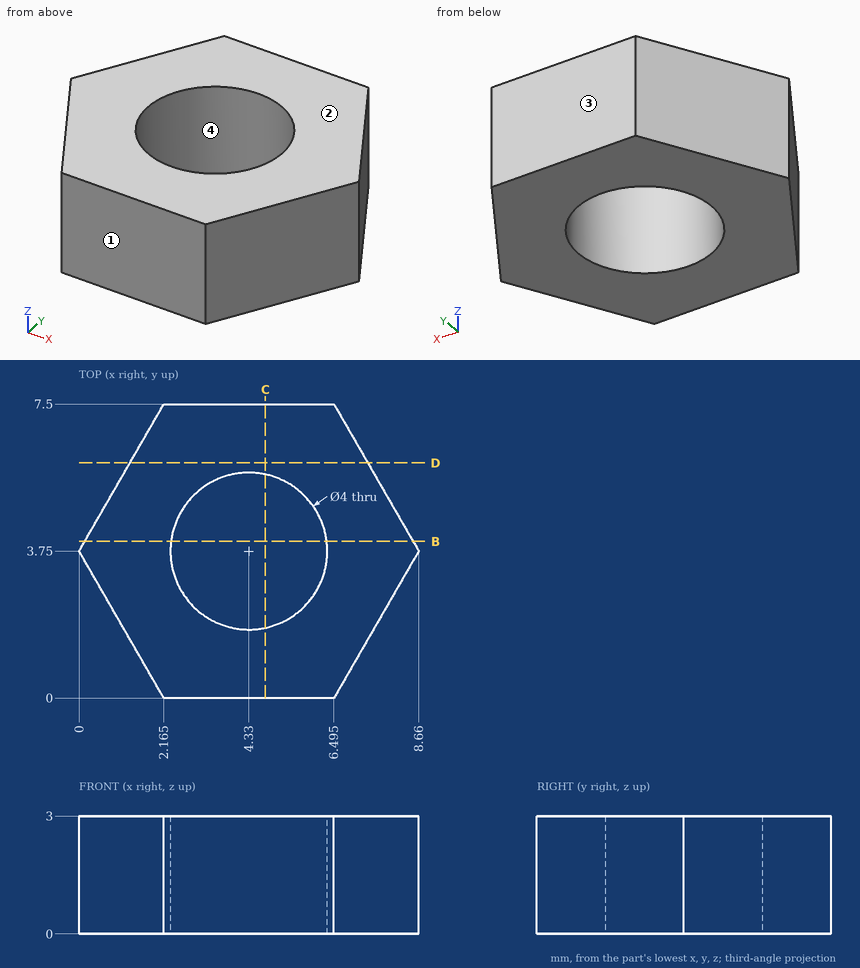
Answer from the drawing. Dimensions are ordinates in mm from the lowest x, y and z of the part. Coordinates: 2 decimals unless noted, no trailing zeros. Order: outer loops, then holes, each group sorted by start corner. A loop starts at its lowest first (then second) coordinate and runs counter-clockwise, first axis right, second up. Notation, with made-up numbers: (32.5, 54) - (83.5, 54) arc R10 cw to (83.5, 65) - close; hole circle Ø4 at (54, 78). An arc over 180 degrees is marked (long way). Put each result on its own line as item: value. Start each with the question number.
1) Find section D-D (y = 6). Give the vertices of the cut face in (x, z), plus the area to 3 significant figures.
2) Find section C-C (x = 4.75). Give the vertices of the cut face in (y, z).
3) A flat-ended cylindrical pin translates along its axis: pin 1 (1.5 mm diameter, centred on y = 5, z = 2.5, fed in from +X). Find the tip coordinate at first contact, or state that the pin passes through.
4) Find section B-B (y = 4). Give the vertices of the cut face in (x, z).
5) For a pull along Y with two mould halves and no side action, classify the marked faces 1, 2, 3 and 4 as released by +Y, released by -Y, zero draft, split by the parting line, or undercut.
6) Find the intervals of material crossed by line 1 (Y direction, x = 4.25, z = 2.35); line 2 (Y direction, x = 3.5, z = 2.05); line 3 (X direction, y = 2.75, z = 0.9), in increasing order. Write a range as from..to.
Results list:
1. outline: (1.3, 0) - (7.36, 0) - (7.36, 3) - (1.3, 3) - close
1. area: 18.2 mm^2
2. outline: (0, 0) - (1.79, 0) - (1.79, 3) - (0, 3) - close; (5.71, 0) - (7.5, 0) - (7.5, 3) - (5.71, 3) - close
3. pin 1: stops at x = 8.37
4. outline: (0.14, 0) - (2.35, 0) - (2.35, 3) - (0.14, 3) - close; (6.31, 0) - (8.52, 0) - (8.52, 3) - (6.31, 3) - close
5. face 1: released by -Y
5. face 2: zero draft
5. face 3: released by +Y
5. face 4: undercut
6. line 1: y = 0..1.75, 5.75..7.5
6. line 2: y = 0..1.93, 5.57..7.5
6. line 3: x = 0.58..2.6, 6.06..8.08
